```python
from build123d import *

# Parameters (mm, degrees)
F0_R     = 12.5
F1_DEPTH = 25.4
F2_DEPTH = 61.722


with BuildPart() as f1:
    # F0 (on Top) → F1 (new body)
    with BuildSketch(Plane.XY):
        with BuildLine():
            ThreePointArc((0.635351, -24.991925), (17.900891, -17.451593), (25, 0))
            ThreePointArc((25, 0), (17.897276, 17.4553), (0.625, 24.992186))
            ThreePointArc((0.625, 24.992186), (-24.999999, -0.005177), (0.635351, -24.991925))
        make_face()
        Circle(F0_R, mode=Mode.SUBTRACT)
        with BuildLine():
            ThreePointArc((0.625, 24.992186), (17.897276, 17.4553), (25, 0))
            ThreePointArc((25, 0), (17.900891, -17.451593), (0.635351, -24.991925))
            Line((0.635351, -24.991925), (99.206847, -22.486016))
            ThreePointArc((99.206847, -22.486016), (77.510213, 0.677835), (100.5625, 22.492968))
            Line((100.5625, 22.492968), (0.625, 24.992186))
        make_face()
        with BuildLine():
            ThreePointArc((122.5, 0), (116.107549, 15.70977), (100.5625, 22.492968))
            ThreePointArc((100.5625, 22.492968), (77.510213, 0.677835), (99.206847, -22.486016))
            ThreePointArc((99.206847, -22.486016), (115.626965, -16.187896), (122.5, 0))
        make_face()
        with Locations((100, 0)):
            Circle(F0_R, mode=Mode.SUBTRACT)
    extrude(amount=F1_DEPTH)

    # F0 (on Top) → F2 (join)
    with BuildSketch(Plane.XY):
        Circle(F0_R)
        Polygon((-2.443647, 2.525975), (-2.443647, 10.170371), (2.427822, 10.170371), (2.427822, 2.525975), (10.520946, 2.525975), (10.520946, -2.345494), (2.427822, -2.345494), (2.427822, -10.938356), (-2.443647, -10.938356), (-2.443647, -2.345494), (-10.587781, -2.345494), (-10.587781, 2.525975), align=None, mode=Mode.SUBTRACT)
    extrude(amount=F2_DEPTH)


solid = f1.part
```
Read the model definition and answer for the solid it produces. Units are mm, in the model's axes. A direction names the side the tool comes from. Coordinates: 2 decimals unless noted, no trailing zeros. Write each loop counter-clockwise with the first axis right and the second up, starting at its lowest first coordinate (ties: lowest second). Pieces come first, ordered by that corner, then holes. Notation, with made-up numbers: (-12.75, 40.25) - (8.25, 40.25) arc R17 cw to (8.25, 69.25) - close; hole circle Ø6 at (-17.5, 36.25). An arc over 180 degrees is marked (long way). Answer as a JSON object with one key per item and string values. Group by question number.
1. A cutting plane is placed at D-D (y = 4.5). Determine the outline of the cut face in (x, z), plus the area to 3 significant figures.
2. Which of the six approach directions +Z, -Z, +X, -X, +Y, -Y give full straight-line access (tool end or side, diameter ignored) to faces 4 (the flat face through (48, 0, 0)), 5 (the flat face through (-6, -2.345, 30))?
3. A cutting plane is placed at A-A (z = 43). Determine the outline of the cut face in (x, y).
4. Each of these flat-tipped pins is pushed along its axis until it touches: P1, Ø6.5, axis at x = -7, z = 32.5, coming from the +Y side; P2, Ø2, axis at x = 11.5, y = -18, coming from the +Z side; P3, Ø4, axis at x = 7.5, z = 27, coming from the -Y side; P4, Ø3, axis at y = 15, z = 54.5, coming from the +X side. Where does it stop, or does it pass through?
5. The mould has two halves that part along X. Classify faces 1 (the flat face through (48, 0, 25.4)), 2 (the flat face through (-2.444, -7, 30)), 3 (the cylindrical face through (11.923, 3.755, 43.307)): +X half, -X half, draft (parallel to the pull), parting line (faces both ways), or undercut.
6. A cutting plane is placed at C-C (z = 5). Determine the outline of the cut face in (x, y) (1 decimal), plus the area to 3 significant figures.
7. A cutting plane is placed at B-B (y = -5.5). Determine the outline of the cut face in (x, z).
8. Consider L1, parallel to Y at x = 100, z = 9; L2, parallel to Z at x = -15, y = -9; L3, parallel to Y at x = 1, z = 13.5. Determine where each line is inside the solid, lowest interval first. Write a range as [from, to].
Worked out:
{
 "1": {"outline": "(-24.59, 0) - (-2.44, 0) - (-2.44, 61.72) - (-11.66, 61.72) - (-11.66, 25.4) - (-24.59, 25.4) - close; (2.43, 0) - (88.34, 0) - (88.34, 25.4) - (11.66, 25.4) - (11.66, 61.72) - (2.43, 61.72) - close; (111.66, 0) - (122.05, 0) - (122.05, 25.4) - (111.66, 25.4) - close", "area": "3,680 mm²"},
 "2": {"face 4": "-Z, +X, -X, +Y, -Y", "face 5": "+Z, -Z"},
 "3": {"outline": "circle Ø25 at (0, 0); hole (-10.59, -2.35) - (-2.44, -2.35) - (-2.44, -10.94) - (2.43, -10.94) - (2.43, -2.35) - (10.52, -2.35) - (10.52, 2.53) - (2.43, 2.53) - (2.43, 10.17) - (-2.44, 10.17) - (-2.44, 2.53) - (-10.59, 2.53) - close"},
 "4": {"P1": "stops at y = 11.92", "P2": "stops at z = 25.4", "P3": "stops at y = -24.85", "P4": "passes through"},
 "5": {"face 1": "draft", "face 2": "undercut", "face 3": "parting line"},
 "6": {"outline": "(0.6, -25) - (99.2, -22.5) arc R22.5 ccw (long way) to (100.6, 22.5) - (0.6, 25) arc R25 ccw (long way) to start; hole (-10.6, -2.3) - (-2.4, -2.3) - (-2.4, -10.9) - (2.4, -10.9) - (2.4, -2.3) - (10.5, -2.3) - (10.5, 2.5) - (2.4, 2.5) - (2.4, 10.2) - (-2.4, 10.2) - (-2.4, 2.5) - (-10.6, 2.5) - close; hole circle Ø25 at (100, 0)", "area": "5,850 mm²"},
 "7": {"outline": "(-24.39, 0) - (-2.44, 0) - (-2.44, 61.72) - (-11.22, 61.72) - (-11.22, 25.4) - (-24.39, 25.4) - close; (2.43, 0) - (88.78, 0) - (88.78, 25.4) - (11.22, 25.4) - (11.22, 61.72) - (2.43, 61.72) - close; (111.22, 0) - (121.82, 0) - (121.82, 25.4) - (111.22, 25.4) - close"},
 "8": {"L1": "y = [-22.5, -12.5], [12.5, 22.51]", "L2": "z = [0, 25.4]", "L3": "y = [-24.98, -10.94], [10.17, 24.98]"}
}
